```python
from build123d import *

# Parameters (mm, degrees)
SKETCH1_W           = 130
SKETCH1_H           = 60
BOSS_EXTRUDE2_DEPTH = 50
SHELL1_T            = -5
CUT_EXTRUDE1_REACH  = 132
SKETCH2_R           = 8.25
SKETCH3_R           = 8.25
CUT_EXTRUDE2_DEPTH  = 61
SKETCH4_W           = 40
SKETCH4_H           = 5
CUT_EXTRUDE3_DEPTH  = 61


with BuildPart() as part:
    # Sketch1 → Boss-Extrude2 (new body)
    with BuildSketch(Plane(origin=(0, 0, 0), x_dir=(1, 0, 0), z_dir=(0, 1, 0))):
        Rectangle(SKETCH1_W, SKETCH1_H)
    extrude(amount=BOSS_EXTRUDE2_DEPTH)

    # Shell1
    shell1_openings = [part.faces().sort_by_distance(p)[0] for p in [
        (0, 50, 0),
    ]]
    offset(amount=SHELL1_T, openings=shell1_openings, kind=Kind.INTERSECTION)

    # Sketch2 → Cut-Extrude1 (cut, up to next)
    with BuildSketch(Plane(origin=(65, 0, 0), x_dir=(0, 0, -1), z_dir=(1, 0, 0)), mode=Mode.PRIVATE) as cut_extrude1_sk1:
        with Locations((-13, 35)):
            Circle(SKETCH2_R)
    cut_extrude1_tool1 = extrude(cut_extrude1_sk1.sketch, amount=-CUT_EXTRUDE1_REACH, mode=Mode.PRIVATE) & part.part
    add(cut_extrude1_tool1.solids().sort_by_distance((65, 35, 13))[0], mode=Mode.SUBTRACT)
    # Sketch2 → Cut-Extrude1 (cut, up to next)
    with BuildSketch(Plane(origin=(65, 0, 0), x_dir=(0, 0, -1), z_dir=(1, 0, 0)), mode=Mode.PRIVATE) as cut_extrude1_sk2:
        with BuildLine():
            ThreePointArc((21.25, 35), (13, 43.25), (4.75, 35))
            ThreePointArc((4.75, 35), (13, 26.75), (21.25, 35))
        make_face()
    cut_extrude1_tool2 = extrude(cut_extrude1_sk2.sketch, amount=-CUT_EXTRUDE1_REACH, mode=Mode.PRIVATE) & part.part
    add(cut_extrude1_tool2.solids().sort_by_distance((65, 35, -13))[0], mode=Mode.SUBTRACT)

    # Sketch3 → Cut-Extrude2 (cut, through all)
    with BuildSketch(Plane.XY.offset(30)):
        with Locations((22.274243645, 35)):
            Circle(SKETCH3_R)
        with Locations((48.274243645, 35)):
            Circle(SKETCH3_R)
    extrude(amount=-CUT_EXTRUDE2_DEPTH, mode=Mode.SUBTRACT)

    # Sketch4 → Cut-Extrude3 (cut, through all)
    with BuildSketch(Plane(origin=(0, 0, -30), x_dir=(-1, 0, 0), z_dir=(0, 0, -1))):
        with Locations((27.140672083, 35)):
            Rectangle(SKETCH4_W, SKETCH4_H)
    extrude(amount=-CUT_EXTRUDE3_DEPTH, mode=Mode.SUBTRACT)


solid = part.part
```
Geometry: final body of the model. Coordinates: model frame, mm. A direction names the side the tool comes from. Coordinates: 2 decimals unless noted, no trailing zeros. Order: outer loops, then holes, each group sorted by start corner. A loop starts at its lowest first (then second) coordinate and runs counter-clockwise, first axis right, second up. Notation, with made-up numbers: M 17.5,68.25 L 64.5,68.25 A25 cw 64.5,99.25 Z; hole C -3.75,-24 d9. An arc over 180 degrees is marked long. Answer in a Markdown table with one row per item. Add a question column.
Q1. Section query C-C on z = -13. Return the cut outline in (x, y).
Q2. Section query B-B on z = 26.5. Return the cut outline in (x, y).
Q3. Section query D-D on x = 4. Return the cut outline in (y, z).
Q4. Section query A-A on x = -19.5. Return the cut outline in (y, z).
Q5. Mould query, pull axis X, two halves, no side actions, for faces 5 (the flat face through (-65, 25, 0)), 6 (the flat face through (-47.141, 35, -28)), 7 (the flat face through (-1, 25, -30)). Classes: released by +X, released by -X, zero draft, split by the parting line, or undercut.
Q6. Reachability of faces 1 (the cylindrical face through (62.535, 41.956, 8.565)), 2 (the flat face through (60, 27, 0)), 3 (the flat face through (-1, 0, 0)), 4 (the flat face through (-27, 37.5, -28)) from +Z, -Z, +X, -X, +Y, -Y: full face, straight path, thin tool, end or side. Return the list, or none.
Q7. Line query: L1, parallel to Z at x = 59, y = 44; L2, parallel to X at y = 13, z = 0; L3, parallel to Y at x = -45.5, z = 12. Output: solid intervals per line, ascending.
Q8. Contact query for a flat-ended pin moving along its axis: P1, Ø1.5, axis at x = -10, z = 21, coming from the +Y side. Output: stop coordinate, or through.
Completed:
| question | item | result |
|---|---|---|
| 1 | outline | M -65,0 L 65,0 L 65,26.75 L 60,26.75 L 60,5 L -60,5 L -60,50 L -65,50 Z; M 60,43.25 L 65,43.25 L 65,50 L 60,50 Z |
| 2 | outline | M -65,0 L 65,0 L 65,50 L -65,50 Z; hole M -47.14,32.5 L -7.14,32.5 L -7.14,37.5 L -47.14,37.5 Z; hole C 22.27,35 d16.5; hole C 48.27,35 d16.5 |
| 3 | outline | M 0,-30 L 50,-30 L 50,-25 L 5,-25 L 5,25 L 50,25 L 50,30 L 0,30 Z |
| 4 | outline | M 0,-30 L 32.5,-30 L 32.5,-25 L 5,-25 L 5,25 L 32.5,25 L 32.5,30 L 0,30 Z; M 37.5,-30 L 50,-30 L 50,-25 L 37.5,-25 Z; M 37.5,25 L 50,25 L 50,30 L 37.5,30 Z |
| 5 | face 5 | released by -X |
| 5 | face 6 | undercut |
| 5 | face 7 | zero draft |
| 6 | face 1 | +X |
| 6 | face 2 | +Y |
| 6 | face 3 | +Z, -Z, +X, -X, -Y |
| 6 | face 4 | +Z, -Z |
| 7 | L1 | z = -30 to -25, 25 to 30 |
| 7 | L2 | x = -65 to -60, 60 to 65 |
| 7 | L3 | y = 0 to 5 |
| 8 | P1 | stops at y = 5 |
